from build123d import *
from OCP.BRepFilletAPI import BRepFilletAPI_MakeChamfer

# Parameters (mm, degrees)
TABAN_FLAN_1_DEPTH      = 135
IZIM10_R                = 4.25
KES_EKSTR_ZYON1_DEPTH   = 10
IZIM11_W                = 140
IZIM11_H                = 64
KES_EKSTR_ZYON2_DEPTH   = 15
PAH1_SIZE               = 30
PAH1_SIZE2              = 17.320508076
KENAR_FLAN_1_DEPTH      = 105
KENAR_FLAN_1_BEND_DEPTH = 105
RADYUS1_R               = 10
IZIM18_R                = 4.5
KES_EKSTR_ZYON3_DEPTH   = 20
RADYUS2_R               = 10


# Sheet-metal steps are written as plain solids
with BuildPart() as part:
    # Çizim1 → Taban-Flanş1 (new body)
    with BuildSketch(Plane.XY):
        with BuildLine():
            Line((0, 0), (0, 36))
            ThreePointArc((0, 36), (2.343145751, 41.656854249), (8, 44))
            Line((8, 44), (102, 44))
            ThreePointArc((102, 44), (107.656854249, 41.656854249), (110, 36))
            Line((110, 36), (110, 0))
            Line((110, 0), (106, 0))
            Line((106, 0), (106, 36))
            ThreePointArc((106, 36), (104.828427125, 38.828427125), (102, 40))
            Line((102, 40), (8, 40))
            ThreePointArc((8, 40), (5.171572875, 38.828427125), (4, 36))
            Line((4, 36), (4, 0))
            Line((4, 0), (0, 0))
        make_face()
    extrude(amount=TABAN_FLAN_1_DEPTH)

    # Çizim10 → Kes-Ekstrüzyon1 (cut)
    with BuildSketch(Plane(origin=(0, 44, 0), x_dir=(1, 0, 0), z_dir=(0, 1, 0))):
        with Locations(Location((23, -111.5, 0), (0, 0, 270))):
            Circle(IZIM10_R)
        with Locations(Location((83, -111.5, 0), (0, 0, 270))):
            Circle(IZIM10_R)
        with Locations(Location((83, -28.5, 0), (0, 0, 270))):
            Circle(IZIM10_R)
        with Locations(Location((23, -28.5, 0), (0, 0, 270))):
            Circle(IZIM10_R)
    extrude(amount=-KES_EKSTR_ZYON1_DEPTH, mode=Mode.SUBTRACT)

    # Çizim11 → Kes-Ekstrüzyon2 (cut)
    with BuildSketch(Plane(origin=(0, 44, 0), x_dir=(1, 0, 0), z_dir=(0, 1, 0))):
        with Locations((55, -70)):
            Rectangle(IZIM11_W, IZIM11_H)
    extrude(amount=-KES_EKSTR_ZYON2_DEPTH, mode=Mode.SUBTRACT)

    # Pah1: one chamfer whose edges measure the first distance from different faces: ONE call of the kernel's chamfer builder (chamfer() names one face for all edges)
    pah1_edges_1 = [part.edges().sort_by_distance(p)[0] for p in [
        (2, 0, 135),
    ]]
    pah1_side_1 = [part.faces().sort_by_distance(p)[0] for p in [
        (2, 0, 67.5),
    ]]
    pah1_edges_2 = [part.edges().sort_by_distance(p)[0] for p in [
        (108, 0, 135),
    ]]
    pah1_side_2 = [part.faces().sort_by_distance(p)[0] for p in [
        (108, 0, 67.5),
    ]]
    pah1 = BRepFilletAPI_MakeChamfer(part.part.solid().wrapped)
    for e in pah1_edges_1:
        pah1.Add(PAH1_SIZE, PAH1_SIZE2, e.wrapped, pah1_side_1[0].wrapped)  # the first distance lies on this face
    for e in pah1_edges_2:
        pah1.Add(PAH1_SIZE, PAH1_SIZE2, e.wrapped, pah1_side_2[0].wrapped)  # the first distance lies on this face
    add(Compound.cast(pah1.Shape()), mode=Mode.REPLACE)

    # Kenar-Flanş1 section (across the edge) → Kenar-Flanş1 (add)
    with BuildSketch(Plane(origin=(0, -4, 0), x_dir=(0, 1, 0), z_dir=(0, 0, 1))):
        with BuildLine():
            Line((-4, 4), (-4, 36))
            Line((-4, 36), (0, 36))
            Line((0, 36), (0, 4))
            ThreePointArc((0, 4), (1.171572875, 1.171572875), (4, 0))
            Line((4, 0), (4, -4))
            ThreePointArc((4, -4), (-1.656854249, -1.656854249), (-4, 4))
        make_face()
    extrude(amount=KENAR_FLAN_1_DEPTH)

    # Kenar-Flanş1 section 2 (across the edge) → Kenar-Flanş1 bend (add)
    with BuildSketch(Plane(origin=(106, -4, 0), x_dir=(0, 1, 0), z_dir=(0, 0, 1))):
        with BuildLine():
            Line((-4, 4), (-4, 36))
            Line((-4, 36), (0, 36))
            Line((0, 36), (0, 4))
            ThreePointArc((0, 4), (1.171572875, 1.171572875), (4, 0))
            Line((4, 0), (4, -4))
            ThreePointArc((4, -4), (-1.656854249, -1.656854249), (-4, 4))
        make_face()
    extrude(amount=KENAR_FLAN_1_BEND_DEPTH)

    # Radyus1
    radyus1_edges = [part.edges().sort_by_distance(p)[0] for p in [
        (-36, -6, 0),
        (-36, -6, 105),
        (70, -6, 0),
        (70, -6, 105),
    ]]
    fillet(radyus1_edges, radius=RADYUS1_R)

    # Çizim18 → Kes-Ekstrüzyon3 (cut)
    with BuildSketch(Plane.XZ.offset(8)):
        with Locations((85, 80)):
            Circle(IZIM18_R)
        with Locations((85, 20)):
            Circle(IZIM18_R)
        with Locations((-21, 80)):
            Circle(IZIM18_R)
        with Locations((-21, 20)):
            Circle(IZIM18_R)
    extrude(amount=-KES_EKSTR_ZYON3_DEPTH, mode=Mode.SUBTRACT)

    # Radyus2
    radyus2_edges = [part.edges().sort_by_distance(p)[0] for p in [
        (108, 17.320508076, 135),
        (2, 17.320508076, 135),
    ]]
    fillet(radyus2_edges, radius=RADYUS2_R)


solid = part.part
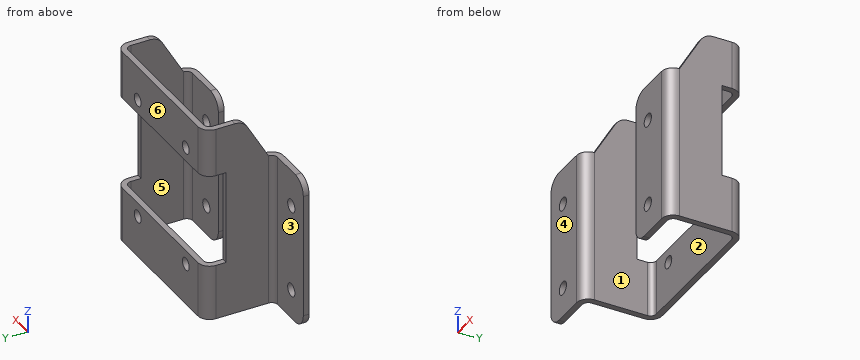
Geometry: final body of the model. Coordinates: model frame, mm. Face numbers are marked on the shaded views. A direction names the side the tool comes from. Coordinates: 2 decimals unless noted, no trailing zeros. Order: outer loops, then holes, each group sorted by start corner. A loop starts at its lowest first (then second) coordinate and runs counter-clockwise, first axis right, second up.
(1) Access query for the marked faces 1, 2 and 3. Directions: +Z, -Z, +X, -X, +Y, -Y. A direction counts if a zero-diameter tool reaches every point of the face in a straight line with its end or side. Return the directions, or none.
(2) Section query C-C (x = 23). Return the cut outline in (y, z), plus the area to 3 significant figures.
(3) Section query D-D (y = 32). Return the cut outline in (x, z), plus the area to 3 significant figures.
(4) First-contact query: pin 1 (7 mm diameter, centred on x = 23, z = 111.5, fed in from -Y); pin 2 (6.5 mm diameter, centred on x = -14, y = -5, fed in from +Z); pin 3 (4.5 mm diameter, centred on x = 2, z = 74.5, fed in from +Y); pin 4 (3 mm diameter, centred on y = 5, z = 49, fed in from -X). Flat tips, straight axial feed; report the tip coordinate or a pass-through.
(5) Section query B-B (z = 80). Return the cut outline in (x, y), plus the area to 3 significant figures.
(6) Material intervals for probe 1 along Z at (x, y) = (-21, -5.1); probe 2 along Z at (x, y) = (101.5, 41.5); probe 3 along X at (y, z) = (6, 42.5), sorted ascending.
(7) Draft query along Y for the marked faces 4, 5 and 6. Return one class per face: pulls with the +Y half, pulls with the -Y half, needs draft (parallel to the pull), parting line crosses it, or undercut.
(8) Section query A-A (x = -21). Return the cut outline in (y, z).
Solution:
1. face 1: +Z, -Z, -Y
1. face 2: +Z, -Z
1. face 3: +Z, -Z, -X, +Y
2. outline: (40, 0) - (44, 0) - (44, 24.25) - (40, 24.25) - close; (40, 32.75) - (44, 32.75) - (44, 38) - (40, 38) - close; (40, 102) - (44, 102) - (44, 107.25) - (40, 107.25) - close; (40, 115.75) - (44, 115.75) - (44, 135) - (40, 135) - close
2. area: 216 mm2
3. outline: (0, 0) - (4, 0) - (4, 38) - (0, 38) - close; (0, 102) - (4, 102) - (4, 135) - (0, 135) - close; (106, 0) - (110, 0) - (110, 38) - (106, 38) - close; (106, 102) - (110, 102) - (110, 135) - (106, 135) - close
3. area: 568 mm2
4. pin 1: passes through
4. pin 2: stops at z = 105
4. pin 3: stops at y = 29
4. pin 4: stops at x = 0
5. outline: (-36, -8) - (-25.5, -8) - (-25.5, -4) - (-36, -4) - close; (-16.5, -8) - (-4, -8) arc R8 ccw to (4, 0) - (4, 29) - (0, 29) - (0, 0) arc R4 cw to (-4, -4) - (-16.5, -4) - close; (70, -8) - (80.5, -8) - (80.5, -4) - (70, -4) - close; (89.5, -8) - (102, -8) arc R8 ccw to (110, 0) - (110, 29) - (106, 29) - (106, 0) arc R4 cw to (102, -4) - (89.5, -4) - close
5. area: 491 mm2
6. probe 1: z = 0 to 15.5, 24.5 to 75.5, 84.5 to 105
6. probe 2: z = 0 to 38, 102 to 135
6. probe 3: x = 0 to 4, 106 to 110
7. face 4: pulls with the -Y half
7. face 5: undercut
7. face 6: pulls with the +Y half
8. outline: (-8, 0) - (-4, 0) - (-4, 15.5) - (-8, 15.5) - close; (-8, 24.5) - (-4, 24.5) - (-4, 75.5) - (-8, 75.5) - close; (-8, 84.5) - (-4, 84.5) - (-4, 105) - (-8, 105) - close
